Source: three-view drawing plus pictorial views. Frame: mm from the lowest corner of the part. A direction names the side the tool comes from. Give positions to 0.01 mm unless a question says otherwise; leave off trailing zeros. Order: outer loops, then holes, each group sorted by start corner. A loop starts at its lowest first (then second) coordinate and runs counter-clockwise, first axis right, second up. Notation, with made-up numbers: (45, 68.5) - (76, 68.5) arc R12 ccw to (76, 72.5) - close; hole circle Ø2 at (14.5, 78.5). An arc over 180 degrees is marked (long way). Answer in a Markdown table with one row per item. Add a question column.
1. Access query for the marked faces 1, 2 and 3. Directions: +Z, -Z, +X, -X, +Y, -Y. A direction counts if a zero-diameter tool reaches every point of the face in a straight line with its end or side. Return the directions, or none.
2. Section query C-C on z = 29.5. Return loops of the section in (x, y), and give its area (3 significant figures).
3. Section query A-A on y = 3.75. Return loops of the section in (x, z), and give its area (3 significant figures).
4. Contact query for flat-ended pins moving along their axis: pin 1 (1.9 mm diameter, centred on y = 4.5, z = 27.5, fed in from -X); pin 2 (1.9 mm diameter, centred on y = 2.5, z = 29.5, fed in from +X). Output: stop coordinate, or through.
5. Section query B-B on x = 40. Return loops of the section in (y, z).
6. Ray query, line 1 (Z direction, x = 44.5, y = 1.75); line 2 (X direction, y = 3.25, z = 25.5). Return the intervals inside material, ascending. Write a range as [from, to].
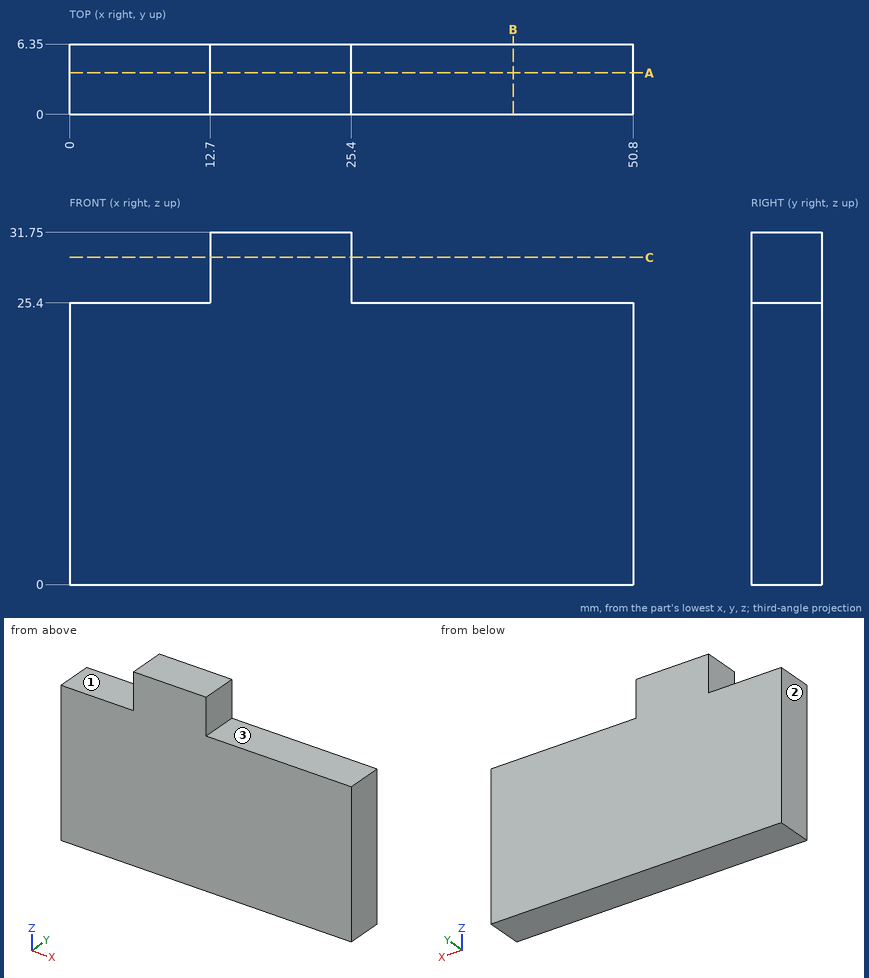
Answer:
| question | item | result |
|---|---|---|
| 1 | face 1 | +Z, -X, +Y, -Y |
| 1 | face 2 | +Z, -Z, -X, +Y, -Y |
| 1 | face 3 | +Z, +X, +Y, -Y |
| 2 | outline | (12.7, 0) - (25.4, 0) - (25.4, 6.35) - (12.7, 6.35) - close |
| 2 | area | 80.6 mm² |
| 3 | outline | (0, 0) - (50.8, 0) - (50.8, 25.4) - (25.4, 25.4) - (25.4, 31.75) - (12.7, 31.75) - (12.7, 25.4) - (0, 25.4) - close |
| 3 | area | 1,370 mm² |
| 4 | pin 1 | stops at x = 12.7 |
| 4 | pin 2 | stops at x = 25.4 |
| 5 | outline | (0, 0) - (6.35, 0) - (6.35, 25.4) - (0, 25.4) - close |
| 6 | line 1 | z = [0, 25.4] |
| 6 | line 2 | x = [12.7, 25.4] |
